Geometry check sheet. Reference: the model listing, model coordinates, mm. A direction names the side the tool comes from. Give positions to 0.01 mm unless a question says otherwise; leave off trailing zeros. Loops run counter-clockwise (first coordinate to the right, second up) from the corner with the lowest first, then second, coordinate; pieces in that order, holes last. Notation, with made-up numbers: (-13, 4.25) -> (16, 4.25) arc R22 cw to (16, 40.25) -> close; hole circle Ø2 at (67.5, -15). An arc over 180 degrees is marked (long way). Answer in a Markdown table with one row per item. Add a question column.
Autodesk Inventor part; units mm, degrees
ref_plane "YZ Plane" through (0, 0, 0) normal (1, 0, 0) x (0, 1, 0)
ref_plane "XZ Plane" through (0, 0, 0) normal (0, 1, 0) x (-1, 0, 0)
ref_plane "XY Plane" through (0, 0, 0) normal (0, 0, 1) x (1, 0, 0)
sketch "Sketch1" plane through (0, 0, 0) normal (1, 0, 0) x (0, 1, 0)
  line L0 (0, 0) -> (25.4, 0)
  line L1 (25.4, 0) -> (25.4, -50.8)
  line L2 (25.4, -50.8) -> (0, -50.8)
  line L3 (0, -50.8) -> (0, 0)
  line L4 (23.8125, -1.5875) -> (1.5875, -1.5875)
  line L5 (1.5875, -1.5875) -> (1.5875, -49.2125)
  line L6 (1.5875, -49.2125) -> (23.8125, -49.2125)
  line L7 (23.8125, -49.2125) -> (23.8125, -1.5875)
  dimension "d0" = 25.4
  dimension "d1" = 50.8
  dimension "d2" = 1.5875
extrude "Extrusion1" add sketch "Sketch1" along normal blind 266.0208
sketch "Sketch2" plane through (0, 25.4, 0) normal (0, 1, 0) x (1, 0, 0)
  line L0 (0, 50.8) -> (0, 0)
  line L1 (0, 0) -> (266.0208, 0)
  line L2 (266.0208, 50.8) -> (266.0208, 0)
  line L3 (0, 50.8) -> (266.0208, 50.8)
  circle A0 centre (12.7, 25.4) radius 3.5687
  circle A1 centre (253.2126, 25.4) radius 3.5687
  point P0 (0, 0)
  dimension "d5" = 7.1374
  dimension "d6" = 12.7
  dimension "d7" = 7.1374
  dimension "d9" = 25.4
  dimension "d10" = 25.4
  dimension "d29" = 240.5126
extrude "Extrusion2" cut sketch "Sketch2" against normal blind 25.4 contours A0 | A1
sketch "Sketch4" plane through (0, 0, 0) normal (0, 0, 1) x (1, 0, 0)
  line L0 (0, 25.4) -> (0, 0)
  line L1 (0, 0) -> (266.0208, 0)
  line L2 (266.0208, 25.4) -> (266.0208, 0)
  line L3 (0, 25.4) -> (266.0208, 25.4)
  line L4 (133.0104, 25.4) -> (133.0104, 0) construction
  circle A0 centre (120.3104, 12.7) radius 2.5781
  circle A1 centre (145.7104, 12.7) radius 2.5781
  dimension "d21" = 5.1562
  dimension "d22" = 5.1562
  dimension "d23" = 12.7
  dimension "d24" = 25.4
  dimension "d27" = 12.7
  dimension "d28" = 12.7
extrude "Extrusion4" cut sketch "Sketch4" against normal through all contours A0 | A1
properties part number "2inTubeBase"
1. Access from +Z, -Z, +X, -X, +Y, -Y to the whole of each face (thin tool, end or side, straight path). Record for faces 4 (the face through (122.69, 11.71, -0.78)), 5 (the face through (131, 1.588, -25)).
2. Sectioned sample at C-C (x = 12.7). Enter the section's corners in (y, z).
3. Release check for a two-part mould opening along Z. For faces 1 (the face through (131, 0, -26)), 2 (the face through (131, 13, 0)), 3 (the face through (10.07, 0.8, -27.81)) record: released by +Z, released by -Z, zero draft, split by the parting line, or undercut.
4. Sectioned sample at A-A (y = 4). Enter the section's corners in (x, z).
5. Sectioned sample at B-B (z = -45). Enter the section's corners in (x, y).
6. Sectioned sample at D-D (x = 91). Enter the section's corners in (y, z), plus the area to 3 significant figures.
7. Material ranges on L1, parallel to X at y = 0.45, z = -25.4; L2, parallel to Y at x = 190, z = -36; L3, parallel to Z at x = 12.7, y = 24.3, recorded low to high. Write a range as from..to.
Response:
| question | item | result |
|---|---|---|
| 1 | face 4 | +Z, -Z |
| 1 | face 5 | +X, -X |
| 2 | outline | (0, -50.8) -> (25.4, -50.8) -> (25.4, -28.97) -> (23.81, -28.97) -> (23.81, -49.21) -> (1.59, -49.21) -> (1.59, -28.97) -> (0, -28.97) -> close; (0, -21.83) -> (1.59, -21.83) -> (1.59, -1.59) -> (23.81, -1.59) -> (23.81, -21.83) -> (25.4, -21.83) -> (25.4, 0) -> (0, 0) -> close |
| 3 | face 1 | zero draft |
| 3 | face 2 | released by +Z |
| 3 | face 3 | undercut |
| 4 | outline | (0, -50.8) -> (266.02, -50.8) -> (266.02, -49.21) -> (0, -49.21) -> close; (0, -1.59) -> (266.02, -1.59) -> (266.02, 0) -> (0, 0) -> close |
| 5 | outline | (0, 0) -> (266.02, 0) -> (266.02, 1.59) -> (0, 1.59) -> close; (0, 23.81) -> (266.02, 23.81) -> (266.02, 25.4) -> (0, 25.4) -> close |
| 6 | outline | (0, -50.8) -> (25.4, -50.8) -> (25.4, 0) -> (0, 0) -> close; hole (1.59, -49.21) -> (23.81, -49.21) -> (23.81, -1.59) -> (1.59, -1.59) -> close |
| 6 | area | 232 mm2 |
| 7 | L1 | x = 0..9.13, 16.27..249.64, 256.78..266.02 |
| 7 | L2 | y = 0..1.59, 23.81..25.4 |
| 7 | L3 | z = -50.8..-28.97, -21.83..0 |
